Build history of the part. All positions in model axes, mm. Face numbers are marked on the shaded views. A direction names the side the tool comes from. Round coordinates to 2 decimals unless told otherwise and drop trailing zeros. Loops run counter-clockwise (first coordinate to the right, second up) from the corner with the lowest first, then second, coordinate; pieces in that order, holes last. Notation, with made-up numbers: (75.25, 32) - (99.25, 32) arc R25 ccw to (99.25, 56) - close; hole circle Ø5 at (88, -11). An arc over 180 degrees is marked (long way). Use a Markdown table: item, result.
from build123d import *

# Parameters (mm, degrees)
SKETCH1_W           = 25.1
SKETCH1_H           = 25.1
BOSS_EXTRUDE1_DEPTH = 0.83
SKETCH2_W           = 25
SKETCH2_H           = 25
BOSS_EXTRUDE2_DEPTH = 5
FILLET1_R           = 5
BOSS_EXTRUDE3_DEPTH = 2.4
CHAMFER1_SIZE       = 0.5


with BuildPart() as part:
    # Sketch1 → Boss-Extrude1 (new body)
    with BuildSketch(Plane(origin=(0, 0, 0), x_dir=(1, 0, 0), z_dir=(0, 1, 0))):
        Rectangle(SKETCH1_W, SKETCH1_H)
    extrude(amount=BOSS_EXTRUDE1_DEPTH)

    # Sketch2 → Boss-Extrude2 (add)
    with BuildSketch(Plane(origin=(0, 0, 0), x_dir=(1, 0, 0), z_dir=(0, 1, 0))):
        Rectangle(SKETCH2_W, SKETCH2_H)
    extrude(amount=BOSS_EXTRUDE2_DEPTH)

    # Fillet1
    fillet1_edges = [part.edges().sort_by_distance(p)[0] for p in [
        (12.5, 2.915, 12.5),
        (12.5, 2.915, -12.5),
        (-12.5, 2.915, -12.5),
        (-12.5, 2.915, 12.5),
    ]]
    fillet(fillet1_edges, radius=FILLET1_R)

    # Sketch3 → Boss-Extrude3 (add)
    with BuildSketch(Plane(origin=(0, 0, 0), x_dir=(1, 0, 0), z_dir=(0, 1, 0))):
        Polygon((8, 7), (-8, 7), (-8, -7), (8, -7), (8, -1.5), (5, -1.5), (5, 1.5), (8, 1.5), align=None)
    extrude(amount=-BOSS_EXTRUDE3_DEPTH)

    # Chamfer1
    chamfer1_edges = [part.edges().sort_by_distance(p)[0] for p in [
        (0, 0, -7),
        (0, 0, 7),
    ]]
    chamfer(chamfer1_edges, length=CHAMFER1_SIZE)


solid = part.part
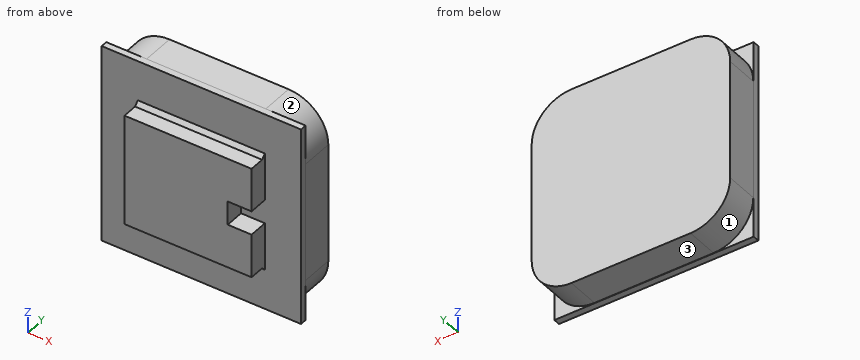
Q1. Drop flat-ended pins along their axis: pin 1 (1.3 mm diameter, centred on y = 2, z = -2.5, fed in from +X); pin 2 (1 mm diameter, centred on x = -4, y = -1.5, fed in from -Z); pin 3 (1.2 mm diameter, centred on y = -1, z = 5, fed in from +X). Give the stop position or say it passes through.
Results found:
| item | result |
|---|---|
| pin 1 | stops at x = 12.5 |
| pin 2 | stops at z = -7 |
| pin 3 | stops at x = 8 |
Q2. Cut at D-D, the plane z = -5.5. List the corners of the cut face in (x, y), plus the area to 3 significant figures.
Results found:
| item | result |
|---|---|
| outline | (-12.55, 0) - (-8, 0) - (-8, -2.4) - (8, -2.4) - (8, 0) - (12.55, 0) - (12.55, 0.83) - (12.5, 0.83) - (12.5, 5) - (-12.5, 5) - (-12.5, 0.83) - (-12.55, 0.83) - close |
| area | 163 mm2 |
Q3. Which spindle directions (+Z, -Z, +X, -X, +Y, -Y) get a long thin tool onto all of the face, cutting with end or side? Do the marked faces 1, 2 and 3. Say none if no direction does.
Results found:
| item | result |
|---|---|
| face 1 | -Z, -X, +Y |
| face 2 | +Z, +X, +Y |
| face 3 | -Z, +X, -X, +Y |
Q4. Probe line 1 (Z direction, x = 3.25, y = -2); line 2 (Z direction, x = -2, y = 3.75); line 3 (Y direction, x = 8, z = -10.75). List the from-to ranges inside material, lowest first.
Results found:
| item | result |
|---|---|
| line 1 | z = -7 to 7 |
| line 2 | z = -12.5 to 12.5 |
| line 3 | y = 0 to 5 |
Q5. Cut at B-B, the plane z = -10.5. List the corners of the cut face in (x, y), plus the area to 3 significant figures.
Results found:
| item | result |
|---|---|
| outline | (-12.55, 0) - (12.55, 0) - (12.55, 0.83) - (11.5, 0.83) - (11.5, 5) - (-11.5, 5) - (-11.5, 0.83) - (-12.55, 0.83) - close |
| area | 117 mm2 |
Q6. Cut at C-C, the plane y = 1.25. List the corners of the cut face in (x, z), plus the area to 3 significant figures.
Results found:
| item | result |
|---|---|
| outline | (-12.5, -7.5) arc R5 ccw to (-7.5, -12.5) - (7.5, -12.5) arc R5 ccw to (12.5, -7.5) - (12.5, 7.5) arc R5 ccw to (7.5, 12.5) - (-7.5, 12.5) arc R5 ccw to (-12.5, 7.5) - close |
| area | 604 mm2 |
Q7. Cut at A-A, the plane x = 1.75. List the corners of the cut face in (y, z), plus the area to 3 significant figures.
Results found:
| item | result |
|---|---|
| outline | (-2.4, -7) - (-0.5, -7) - (0, -7.5) - (0, -12.55) - (0.83, -12.55) - (0.83, -12.5) - (5, -12.5) - (5, 12.5) - (0.83, 12.5) - (0.83, 12.55) - (0, 12.55) - (0, 7.5) - (-0.5, 7) - (-2.4, 7) - close |
| area | 159 mm2 |
